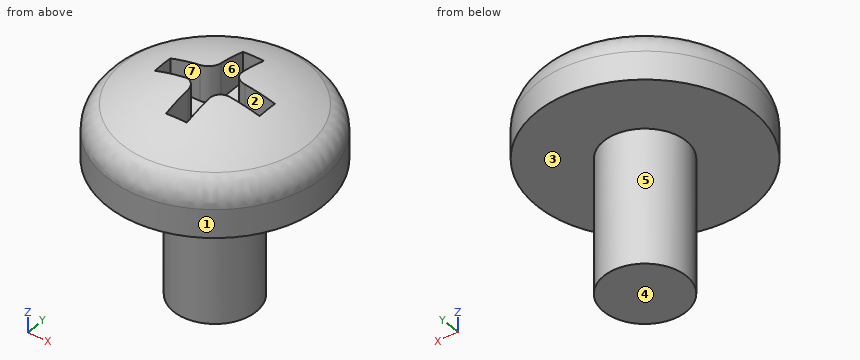
from build123d import *

# Parameters (mm, degrees)
F0_R     = 1.7526
F1_DEPTH = 5.715
F4_R     = 1.27
F7_DEPTH = 2.921
F8_R     = 0.508


with BuildPart() as f1:
    # F0 (on Top) → F1 (new body)
    with BuildSketch(Plane.XY):
        Circle(F0_R)
    extrude(amount=F1_DEPTH)

    # F2 (on Right) → F3 (revolve)
    with BuildSketch(Plane.YZ):
        with BuildLine():
            Line((-4.5974, 7.62), (-4.5974, 5.715))
            Line((-4.5974, 5.715), (0, 5.715))
            Line((0, 5.715), (0, 9.0932))
            ThreePointArc((0, 9.0932), (-2.4088, 8.700189), (-4.5974, 7.62))
        make_face()
    revolve(axis=Axis((0, 0, 4.5466), (0, 0, 1)))

    # F4
    f4_edges = [f1.edges().sort_by_distance(p)[0] for p in [
        (0, 4.5974, 7.62),
    ]]
    fillet(f4_edges, radius=F4_R)

    # F6 (on offset) → F7 (cut)
    with BuildSketch(Plane.XY.offset(10.414)):
        Polygon((-2.2225, 0.4445), (-2.2225, -0.4445), (-0.4445, -0.4445), (-0.4445, -2.2225), (0.4445, -2.2225), (0.4445, -0.4445), (2.2225, -0.4445), (2.2225, 0.4445), (0.4445, 0.4445), (0.4445, 2.2225), (-0.4445, 2.2225), (-0.4445, 0.4445), align=None)
    extrude(amount=-F7_DEPTH, mode=Mode.SUBTRACT)

    # F8
    f8_edges = [f1.edges().sort_by_distance(p)[0] for p in [
        (-0.4445, 0.4445, 8.276901),
        (0.4445, 0.4445, 8.276901),
        (-0.4445, -0.4445, 8.276901),
        (0.4445, -0.4445, 8.276901),
    ]]
    fillet(f8_edges, radius=F8_R)


solid = f1.part
Work out the finished part from the listing and answer in its coordinate system (mm). Face numbers are marked on the shaded views. A direction names the side the tool comes from. Round coordinates to 2 decimals unless told otherwise and drop trailing zeros. Write each loop counter-clockwise with the first axis right and the second up, starting at its lowest first coordinate (ties: lowest second). Pieces come first, ordered by that corner, then holes. Notation, with made-up numbers: (68, -28) - (116, -28) arc R22 ccw to (116, -22) - close; hole circle Ø10 at (0.25, 17). An arc over 180 degrees is marked (long way). Answer in a Markdown table with one row per item. Add a question column.
1. A cutting plane is placed at A-A, the plane z = 1.25. Determine the outline of the cut face in (x, y).
2. The mould has two halves that part along Y. Classify the marked faces 4, 5, 6 and 7: +Y half, -Y half, draft (parallel to the pull), parting line (faces both ways), or undercut.
3. Find the intervals of material crossed by line 1 along Z through (x, y) = (-1.25, 0); line 2 along Z through (x, y) = (0.75, -0.75); line 3 along X through (y, z) = (1.25, 2.5), in increasing order. Write a range as from..to.
4. Given pin 1 (1.5 mm diameter, centred on y = 2, z = 3, fed in from -X); pin 2 (1 mm diameter, centred on y = -1.5, z = 8, fed in from +X); pin 3 (0.7 mm diameter, centred on x = 0, z = 8, fed in from -Y), each flat-ended and moving along its own axis, determine where each tip first touches the part or whether it passes through.
5. For the marked faces 1, 2 and 3, determine the directions among +Z, -Z, +X, -X, +Y, -Y from which every point of the face is accessible in a straight line to the end or side of a thin tool.
Worked out:
| question | item | result |
|---|---|---|
| 1 | outline | circle Ø3.51 at (0, 0) |
| 2 | face 4 | draft |
| 2 | face 5 | parting line |
| 2 | face 6 | undercut |
| 2 | face 7 | undercut |
| 3 | line 1 | 0..7.49 |
| 3 | line 2 | 0..9.01 |
| 3 | line 3 | -1.23..1.23 |
| 4 | pin 1 | x = -1.23 |
| 4 | pin 2 | x = 4.24 |
| 4 | pin 3 | y = -4.37 |
| 5 | face 1 | +Z, -Z |
| 5 | face 2 | +Z |
| 5 | face 3 | -Z |
